The listing builds one solid part. Answer for the finished solid, in the listing's coordinates (mm). A direction names the side the tool comes from. Round coordinates to 2 decimals unless told otherwise and drop trailing zeros. Order: outer loops, then holes, each group sorted by start corner. A loop starts at its lowest first (then second) coordinate and runs counter-clockwise, first axis right, second up. Notation, with made-up numbers: (20.5, 32.25) -> (58.5, 32.25) arc R10 cw to (58.5, 38.25) -> close; hole circle Ø8 at (42, 50.5). An arc over 180 degrees is marked (long way). Return JSON: item names as keys, results as strings. Group by question number.
(1) The part is cut by section C-C (x = 88). Determine the outline of the cut face in (y, z), plus the area to 3 significant figures.
(2) Consider line 1 (Z direction, x = 65, y = 3.9); line 2 (X direction, y = 2.1, z = -6); line 3 (X direction, y = 0.3, z = -79). Determine where each line is inside the solid, lowest interval first. Write a range as [from, to].
(3) Which of the six approach directions +Z, -Z, +X, -X, +Y, -Y give full straight-line access (tool end or side, diameter ignored) to faces 4 (the face through (88, 2, -85)), 5 (the face through (100, 2, -71))?
(4) The part is cut by section A-A (x = 6). Determine the outline of the cut face in (y, z), plus the area to 3 significant figures.
(5) Determine the mould class of faces 1 (the face through (66.43, 2.54, -6.45)), 2 (the face through (49, 2, 0)), 3 (the face through (49, 5, -73)) for opening direction Z: +Z half, -Z half, draft (parallel to the pull), parting line (faces both ways), or undercut.
(6) The part is cut by section B-B (z = -138). Determine the outline of the cut face in (x, y), plus the area to 3 significant figures.
from build123d import *

# Parameters (mm, degrees)
SKETCH1_W           = 100
SKETCH1_H           = 144
BOSS_EXTRUDE1_DEPTH = 5
SKETCH2_R           = 1.5
CUT_EXTRUDE1_DEPTH  = 6


with BuildPart() as part:
    # Sketch1 → Boss-Extrude1 (new body)
    with BuildSketch(Plane(origin=(0, 0, 0), x_dir=(1, 0, 0), z_dir=(0, 1, 0))):
        with Locations((50, 72)):
            Rectangle(SKETCH1_W, SKETCH1_H)
        with BuildLine():
            Line((85, 82), (85, 62))
            ThreePointArc((85, 62), (88, 59), (91, 62))
            Line((91, 62), (91, 82))
            ThreePointArc((91, 82), (88, 85), (85, 82))
        make_face(mode=Mode.SUBTRACT)
    extrude(amount=BOSS_EXTRUDE1_DEPTH)

    # Sketch2 → Cut-Extrude1 (cut, through all)
    with BuildSketch(Plane(origin=(0, 5, 0), x_dir=(1, 0, 0), z_dir=(0, 1, 0))):
        with Locations((6, 138)):
            Circle(SKETCH2_R)
        with Locations((6, 6)):
            Circle(SKETCH2_R)
        with Locations((65, 138)):
            Circle(SKETCH2_R)
        with Locations((65, 6)):
            Circle(SKETCH2_R)
    extrude(amount=-CUT_EXTRUDE1_DEPTH, mode=Mode.SUBTRACT)


solid = part.part
Answer below:
{
 "1": {"outline": "(0, -144) -> (5, -144) -> (5, -85) -> (0, -85) -> close; (0, -59) -> (5, -59) -> (5, 0) -> (0, 0) -> close", "area": "590 mm²"},
 "2": {"line 1": "z = [-144, -139.5], [-136.5, -7.5], [-4.5, 0]", "line 2": "x = [0, 4.5], [7.5, 63.5], [66.5, 100]", "line 3": "x = [0, 85], [91, 100]"},
 "3": {"face 4": "+Y, -Y", "face 5": "+Z, -Z, +X, +Y, -Y"},
 "4": {"outline": "(0, -144) -> (5, -144) -> (5, -139.5) -> (0, -139.5) -> close; (0, -136.5) -> (5, -136.5) -> (5, -7.5) -> (0, -7.5) -> close; (0, -4.5) -> (5, -4.5) -> (5, 0) -> (0, 0) -> close", "area": "690 mm²"},
 "5": {"face 1": "undercut", "face 2": "+Z half", "face 3": "draft"},
 "6": {"outline": "(0, 0) -> (4.5, 0) -> (4.5, 5) -> (0, 5) -> close; (7.5, 0) -> (63.5, 0) -> (63.5, 5) -> (7.5, 5) -> close; (66.5, 0) -> (100, 0) -> (100, 5) -> (66.5, 5) -> close", "area": "470 mm²"}
}
